from build123d import *

# Parameters (mm, degrees)
F0_R     = 8
F0_R_2   = 5.1
F0_R_3   = 4.1
F1_DEPTH = 4.7
F2_DEPTH = 24.7
F3_R     = 0.3
F4_R     = 0.75


with BuildPart() as f1:
    # F0 (on Top) → F1 (new body)
    with BuildSketch(Plane.XY):
        Circle(F0_R)
        Circle(F0_R_2, mode=Mode.SUBTRACT)
        Circle(F0_R_2)
        Circle(F0_R_3, mode=Mode.SUBTRACT)
        Circle(F0_R_3)
    extrude(amount=F1_DEPTH)

    # F0 (on Top) → F2 (join)
    with BuildSketch(Plane.XY):
        Circle(F0_R_2)
        Circle(F0_R_3, mode=Mode.SUBTRACT)
    extrude(amount=F2_DEPTH)

    # F3
    f3_edges = [f1.edges().sort_by_distance(p)[0] for p in [
        (-5.1, 0, 24.7),
        (-4.1, 0, 24.7),
    ]]
    fillet(f3_edges, radius=F3_R)

    # F4
    f4_edges = [f1.edges().sort_by_distance(p)[0] for p in [
        (-8, 0, 0),
    ]]
    fillet(f4_edges, radius=F4_R)


solid = f1.part
Design review of the part built by this model. Coordinates are the model's own, in mm. A direction names the side the tool comes from. Give positions to 0.01 mm unless a question says otherwise; leave off trailing zeros. Order: outer loops, then holes, each group sorted by start corner. A loop starts at its lowest first (then second) coordinate and runs counter-clockwise, first axis right, second up. Notation, with made-up numbers: (-39.75, 20) - (14.25, 20) arc R35 cw to (14.25, 53) - close; hole circle Ø9 at (39.5, 0.5). An arc over 180 degrees is marked (long way). Use CSV: the item, a comma, the result in double quotes. Start each with the question number.
Q1. For line 1 (X direction, y = 0, z = 19); line 2 (Y direction, x = -1, z = 19.5), list the stretches that pass through material, from the lowest coordinate up.
Q2. For P1, Ø5, axis at y = -4, z = 5.5, coming from the +X side; P2, Ø5, axis at x = 0, y = 0, coming from the +Z side; P3, Ø4, axis at y = -5.5, z = 19, coming from the +X side, all flat-tipped, find the tip position at first contact; note any pin that passes through.
Q3. Take a section at A-A (x = 0). State the section outline as (y, z) points.
Q4. Draft analysis for pull direction X (two halves, no side actions). For faces 1 (the face through (0, 0, 0)), 2 (the face through (2.4, -4.5, 14.4)), 3 (the face through (-0.534, 4.065, 14.412)), state which applies: pulls with the +X half, pulls with the -X half, needs draft (parallel to the pull), parting line crosses it, or undercut.
Q5. Take a section at B-B (z = 22). State the section outline as (x, y) points.
Q6. Machinability: for faces 4 (the face through (-1.73, -7.81, 2.7)), 5 (the face through (0, 0, 4.7)), which of the approach directions +Z, -Z, +X, -X, +Y, -Y give a long, thin tool a straight path to every point of the face, cutting with its end or side? Answer none if there is none.
Calculated:
1,line 1,"x = -5.1 to -4.1, 4.1 to 5.1"
1,line 2,"y = -5 to -3.98, 3.98 to 5"
2,P1,"stops at x = 7.83"
2,P2,"stops at z = 4.7"
2,P3,"stops at x = 3.71"
3,outline,"(-8, 0.75) arc R0.75 ccw to (-7.25, 0) - (7.25, 0) arc R0.75 ccw to (8, 0.75) - (8, 4.7) - (5.1, 4.7) - (5.1, 24.4) arc R0.3 ccw to (4.8, 24.7) - (4.4, 24.7) arc R0.3 ccw to (4.1, 24.4) - (4.1, 4.7) - (-4.1, 4.7) - (-4.1, 24.4) arc R0.3 ccw to (-4.4, 24.7) - (-4.8, 24.7) arc R0.3 ccw to (-5.1, 24.4) - (-5.1, 4.7) - (-8, 4.7) - close"
4,face 1,"needs draft"
4,face 2,"parting line crosses it"
4,face 3,"undercut"
5,outline,"circle Ø10.2 at (0, 0); hole circle Ø8.2 at (0, 0)"
6,face 4,"+Z, -Z"
6,face 5,"+Z"
